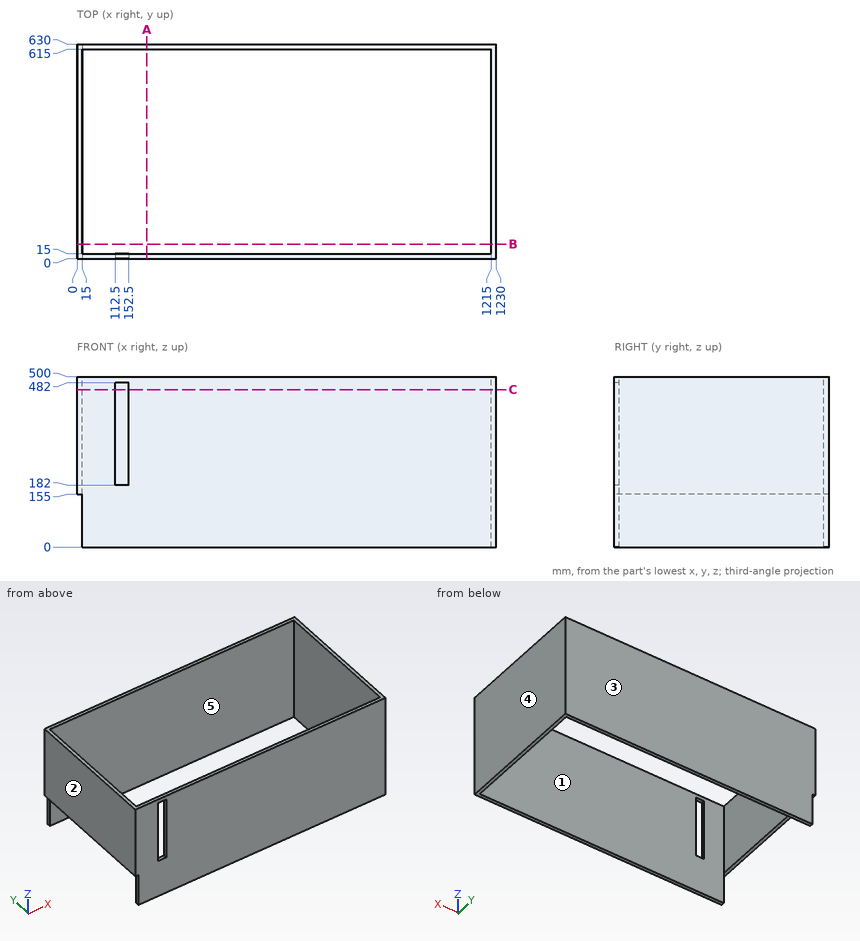
Design review of the part shown in the three views and the two pictorial views. Dimensions are in mm from the part's minimum x, y and z. A direction names the side the tool comes from. Coordinates: 2 decimals unless noted, no trailing zeros. Order: outer loops, then holes, each group sorted by start corner. A loop starts at its lowest first (then second) coordinate and runs counter-clockwise, first axis right, second up. Notation, with made-up numbers: (12.25, 49.5) -> (28.25, 49.5) arc R13 ccw to (28.25, 69.5) -> close; hole circle Ø9 at (36.25, 42.25). An arc over 180 degrees is marked (long way). Use one line per item in the form item = value. Start each with the question number.
(1) Insertion check: pin 1 (12 mm diameter, centred on y = 621.5, z = 68.5, fed in from -X); pin 2 (7.5 mm diameter, centred on x = 4, y = 299.5, fed in from -Z). Each pin has a flat end and moves straight along its axis. Give the tip position at first contact, or say it passes through.
(2) Add section A-A on x = 205. State the section outline as (y, z) points, plus the area to 3 significant figures.
(3) For probe 1 along X at (y, z) = (136, 286); probe 2 along Y at (x, z) = (1035.5, 444); probe 3 along X at (y, z) = (234, 57), list the stretches that pass through material, from the lowest coordinate up.
(4) The part is to be moulded in two halves that separate along X. For the marked faces 1, 2 and 3, say which applies: +X half, -X half, draft (parallel to the pull), parting line (faces both ways), or undercut.
(5) Add section C-C on z = 462. State the section outline as (x, y) points, plus the area to 3 significant figures.
(6) For the marked faces 4 and 5, list the 3-axis set-ups (+Z, -Z, +X, -X, +Y, -Y) from which the entire face can be reached by the end or side of a thin tool; tool diameter is ignored.
(7) Add section B-B on y = 43. State the section outline as (x, z) points.
Answer block:
q1.pin_1 = 15
q1.pin_2 = 155
q2.outline = (0, 0) -> (15, 0) -> (15, 500) -> (0, 500) -> close; (615, 0) -> (630, 0) -> (630, 500) -> (615, 500) -> close
q2.area = 15,000 mm²
q3.probe_1 = 0 to 15, 1215 to 1230
q3.probe_2 = 0 to 15, 615 to 630
q3.probe_3 = 1215 to 1230
q4.face_1 = undercut
q4.face_2 = -X half
q4.face_3 = draft
q5.outline = (0, 0) -> (112.5, 0) -> (112.5, 15) -> (15, 15) -> (15, 615) -> (1215, 615) -> (1215, 15) -> (152.5, 15) -> (152.5, 0) -> (1230, 0) -> (1230, 630) -> (0, 630) -> close
q5.area = 54,300 mm²
q6.face_4 = +Z, -Z, +X, +Y, -Y
q6.face_5 = +Z, -Z
q7.outline = (0, 155) -> (15, 155) -> (15, 500) -> (0, 500) -> close; (1215, 0) -> (1230, 0) -> (1230, 500) -> (1215, 500) -> close
